from build123d import *

# Parameters (mm, degrees)
F0_R           = 50
F1_DEPTH       = 50
F1_TAPER       = 30
F3_D           = 11
F3_DEPTH       = 20
F3_CBORE_D     = 17.25
F3_CBORE_DEPTH = 10
F3_TIP         = 3.3047334047


with BuildPart() as f1:
    # F0 (on Front) → F1 (new body, symmetric)
    with BuildSketch(Plane.XZ):
        Circle(F0_R)
    extrude(amount=F1_DEPTH, both=True, taper=F1_TAPER)

    # F3
    with Locations(Plane.XZ.offset(50)):
        with Locations((0, 0)):
            CounterBoreHole(F3_D / 2, F3_CBORE_D / 2, F3_CBORE_DEPTH, depth=F3_DEPTH)
            with Locations((0, 0, -(F3_DEPTH + F3_TIP / 2))):  # 118° drill point
                Cone(0, F3_D / 2, F3_TIP, mode=Mode.SUBTRACT)


solid = f1.part
Source: CAD feature listing. Evaluate the final solid. Frame: model axes, mm. A direction names the side the tool comes from. Round coordinates to 2 decimals unless told otherwise and drop trailing zeros. Loops run counter-clockwise (first coordinate to the right, second up) from the corner with the lowest first, then second, coordinate; pieces in that order, holes last.
Q1. Ray query, line 1 (Z direction, x = 0, y = -32); line 2 (Z direction, x = 0, y = -46.5) (3 decimals); line 3 (X direction, y = -36, z = 0). Return the intervals inside material, ascending.
Q2. Access query for faces 4 (the face through (1.19, -34.93, -5.37)), 5 (the face through (9, -50, 0)). Directions: +Z, -Z, +X, -X, +Y, -Y. A direction counts if a zero-diameter tool reaches every point of the face in a straight line with its end or side. Return the directions, or none.
Q3. First-contact query: P1, Ø12, axis at y = 26, z = 19, coming from the +X side; P2, Ø2, axis at x = 7.5, z = 31, coming from the -Y side; P3, Ø1.5, axis at x = 27, y = 2, coming from the -Z side. Flat tips, straight axial feed; report the tip coordinate or a pass-through.
Q4. Section A-A, the plane y = -25. Return loops of the section in (x, z).
Q5. Mould query, pull axis Z, two halves, no side actions, for faces 1 (the face through (0, -40, -6)), 2 (the face through (24.55, 42.02, 7.73)), 3 (the face through (0, 50, 0)). Classes: pulls with the +Z half, pulls with the -Z half, needs draft (parallel to the pull), parting line crosses it, or undercut.
Solutions:
1. line 1: z = -31.52 to -5.5, 5.5 to 31.52
1. line 2: z = -23.153 to -8.625, 8.625 to 23.153
1. line 3: x = -29.22 to -5.5, 5.5 to 29.22
2. face 4: -Y
2. face 5: +Z, -Z, +X, -X, -Y
3. P1: stops at x = 34.48
3. P2: stops at y = -33.09
3. P3: stops at z = -41.42
4. outline: circle Ø71.13 at (0, 0)
5. face 1: undercut
5. face 2: parting line crosses it
5. face 3: needs draft
